Autodesk Inventor part; units mm, degrees
ref_plane "Plano de trabajo2" through (-28, -13.5, 0) normal (0, -1, 0) x (1, 0, 0)
ref_plane "YZ Plane" through (0, 0, 0) normal (1, 0, 0) x (0, 1, 0)
ref_plane "XZ Plane" through (0, 0, 0) normal (0, 1, 0) x (-1, 0, 0)
sketch "Boceto1" plane through (0, 0, 0) normal (0, 0, 1) x (1, 0, 0)
  line L0 (-28, -17.5) -> (28, -17.5)
  line L1 (28, -17.5) -> (28, 9.5)
  line L2 (20, 17.5) -> (-20, 17.5)
  line L3 (-28, 9.5) -> (-28, -17.5)
  line L4 (-28, -17.5) -> (28, 17.5) construction
  line L5 (28, -17.5) -> (-28, 17.5) construction
  arc A0 (-20, 17.5) -> (-28, 9.5) centre (-20, 9.5) ccw
  arc A1 (28, 9.5) -> (20, 17.5) centre (20, 9.5) ccw
  circle A2 centre (-20, 9.5) radius 4
  circle A3 centre (20, 9.5) radius 4
  point P0 (0, 0)
  dimension "d0" = 56
  dimension "d1" = 35
  dimension "d2" = 8
  dimension "d3" = 8
  dimension "d4" = 8
extrude "Extrusión1" add sketch "Boceto1" along normal blind 10
ref_plane "Plano de trabajo2" through (-28, -13.5, 0) normal (0, -1, 0) x (1, 0, 0)
sketch "Boceto2" plane through (-28, -13.5, 0) normal (0, -1, 0) x (1, 0, 0)
  circle A0 centre (28.3324, 69.928) radius 15
  circle A1 centre (28.3324, 69.928) radius 10
  line L0 (8, 10) -> (0, 10)
  line L1 (0, 10) -> (13.6726, 73.1043)
  line L2 (56, 0) -> (56, 10)
  line L3 (56, 10) -> (43.0236, 72.9561)
  line L4 (0, 10) -> (56, 10)
  point P0 (28, 0)
  dimension "d8" = 30
  dimension "d9" = 20
extrude "Extrusión2" add sketch "Boceto2" against normal blind 7 contours A0 L3 L4 L0 L1
extrude "Extrusión3" add sketch "Boceto2" against normal blind 11 contours A0
extrude "Extrusión4" add sketch "Boceto2" along normal blind 4 contours A0
sketch "Boceto3" plane through (0, 0, 0) normal (1, 0, 0) x (0, 1, 0)
  line L0 (9.5, 10) -> (-6.5, 10)
  line L1 (-6.5, 10) -> (17.5, 10)
  line L2 (17.5, 10) -> (-2.5, 54.928)
  line L3 (-17.5, 54.928) -> (-2.5, 54.928)
  line L4 (-6.5, 54.928) -> (-6.5, 10)
  line L5 (-6.5, 10) -> (-6.5, 73.1043)
  line L6 (-6.5, 54.928) -> (-2.5, 54.928)
  line L7 (-6.5, 54.928) -> (-6.5, 10)
  point P0 (0, 0)
  dimension "d17" = 24
extrude "Extrusión5" add sketch "Boceto3" along normal mid plane 6
properties part number "Soporte polea"
CAD build for the part. Positions are in the model's coordinates, mm. A direction names the side the tool comes from. Coordinates: 2 decimals unless noted, no trailing zeros. Write each loop counter-clockwise with the first axis right and the second up, starting at its lowest first coordinate (ties: lowest second). Pieces come first, ordered by that corner, then holes.
(1) Cut at C-C, the plane y = -10. List the corners of the cut face in (x, z), and give its area (3 significant figures).
(2) Cut at D-D, the plane y = 10.5. List the corners of the cut face in (x, z).
(3) Cut at A-A, the plane z = 64.5. List the corners of the cut face in (x, y), and give its area (3 significant figures).
(4) Drill centre lines: probe 1 along Z at (x, y) = (0, -14.5); probe 2 along X at (y, z) = (9, 6); probe 3 along Y at (x, z) = (-20, 5.5). Where is each one in solid material? Low to high.
(5) 3-axis set-ups, long thin cutter, end or side, ignore diameter. For faces 5 (the face through (0, -15, 10)), 6 (the face through (3, 3, 28)), 7 (the face through (3, -2.5, 60)): which of +Z, -Z, +X, -X, +Y, -Y reach the whole face in a straight line?
(6) Flat gauge pins, fed straight in: pin 1 (4 mm diameter, centred on y = -11.5, z = 43, fed in from +X); pin 2 (8 mm diameter, centred on x = 19.5, y = 9, fed in from +Z); pin 3 (10 mm diameter, centred on x = 5.5, y = 2, fed in from -Z); pin 4 (1 mm diameter, centred on y = -7.5, z = 42, fed in from -X) (3 decimals). Where does each tip first touch, or does it go through?
(7) Two-plate mould, pull along Y, no slides. Class faces 1 (the face through (-25.719, 15.094, 4.93)), 2 (the face through (-16, 6, 10)), 3 (the face through (-23.2, 11.9, 4.9)), 4 (the face through (16.8, 11.9, 4.9)): +Y half, -Y half, draft (parallel to the pull), parting line (faces both ways), or undercut.
(8) Cut at B-B, the plane x = 5.5. List the corners of the cut face in (y, z), and give its area (3 significant figures).
Geometry says:
1. outline: (-28, 0) - (28, 0) - (28, 10) - (15.02, 72.96) arc R15 ccw to (-14.33, 73.1) - (-28, 10) - close; hole circle Ø20 at (0.33, 69.93)
1. area: 3,200 mm2
2. outline: (-27.94, 0) - (-23.87, 0) - (-23.87, 10) - (-27.94, 10) - close; (-16.13, 0) - (16.13, 0) - (16.13, 10) - (3, 10) - (3, 25.72) - (-3, 25.72) - (-3, 10) - (-16.13, 10) - close; (23.87, 0) - (27.94, 0) - (27.94, 10) - (23.87, 10) - close
3. outline: (-16.19, -13.5) - (-13.65, -13.5) - (-13.65, -17.5) - (-8.07, -17.5) - (-8.07, -2.5) - (-13.65, -2.5) - (-13.65, -6.5) - (-16.19, -6.5) - close; (8.73, -17.5) - (14.32, -17.5) - (14.32, -13.5) - (16.77, -13.5) - (16.77, -6.5) - (14.32, -6.5) - (14.32, -2.5) - (8.73, -2.5) - close
3. area: 202 mm2
4. probe 1: z = 0 to 10, 54.93 to 59.93, 79.92 to 84.92
4. probe 2: x = -28 to -23.97, -16.03 to 16.03, 23.97 to 28
4. probe 3: y = -17.5 to 5.5, 13.5 to 17.5
5. face 5: +X, -X, -Y
5. face 6: +X, +Y
5. face 7: +Z, +X, -X, +Y
6. pin 1: stops at x = 21.61
6. pin 2: stops at z = 10
6. pin 3: stops at z = 0
6. pin 4: stops at x = -21.175
7. face 1: +Y half
7. face 2: draft
7. face 3: undercut
7. face 4: undercut
8. outline: (-17.5, 0) - (17.5, 0) - (17.5, 10) - (-6.5, 10) - (-6.5, 55.85) - (-2.5, 55.85) - (-2.5, 61.37) - (-17.5, 61.37) - (-17.5, 55.85) - (-13.5, 55.85) - (-13.5, 10) - (-17.5, 10) - close; (-17.5, 78.49) - (-2.5, 78.49) - (-2.5, 84.01) - (-17.5, 84.01) - close
8. area: 837 mm2
